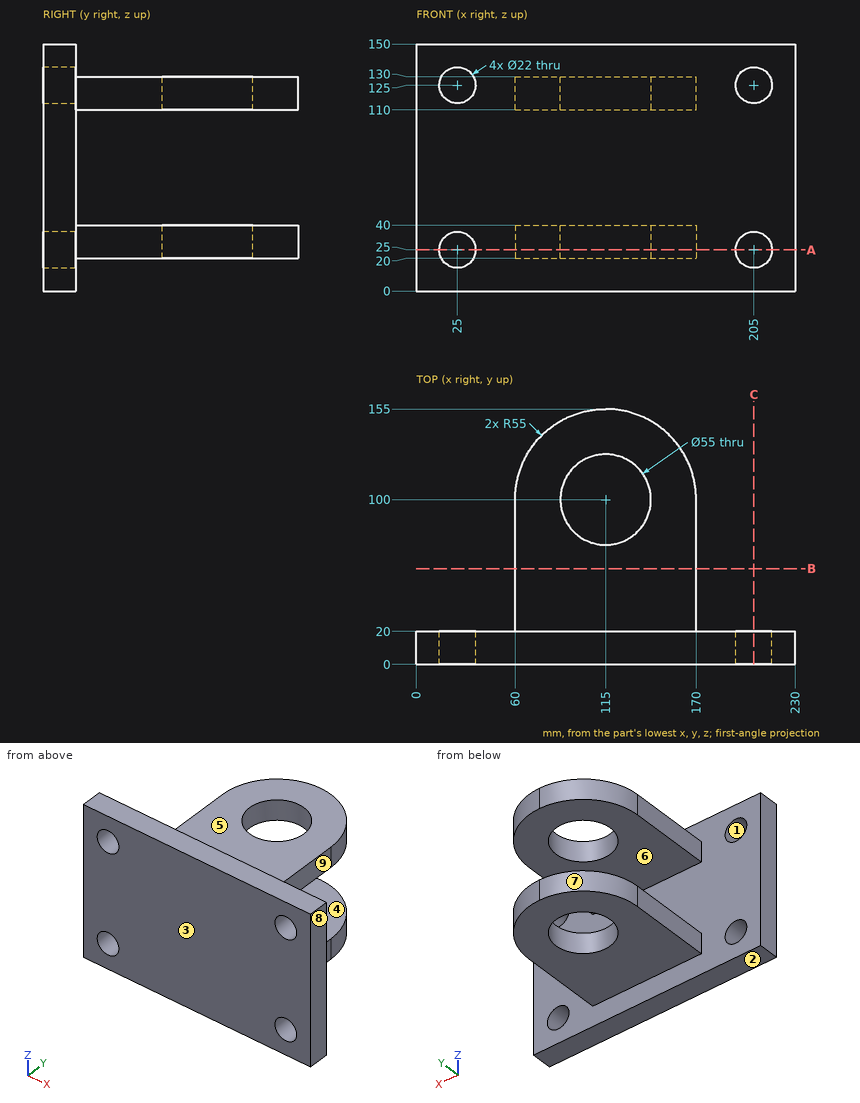
Answer from the drawing. Dimensions are ordinates in mm from the lowest x, y and z of the part. A direction names the side the tool comes from. Give positions to 0.01 mm unless a question says otherwise; leave off trailing zeros. Write each loop counter-clockwise with the first axis right and the second up, starting at its lowest first coordinate (ties: lowest second). Pieces come first, ordered by that corner, then holes. Notation, with made-up numbers: (70.5, 70) - (93.5, 70) arc R37 ccw to (93.5, 108) - close; hole circle Ø7 at (22, 53.5). An arc over 180 degrees is marked (long way). Answer in a Markdown table with one row per item. Add a question column.
Item 1: Section B-B, the plane y = 58 is taken. Write down the section's boundary in (x, z).
Item 2: Find the intervals of material crossed by L1, parallel to X at y = 10, z = 25; L2, parallel to Y at x = 116, z = 29.5; L3, parallel to Z at x = 68, y = 114.5, in increasing order.
Item 3: Section C-C, the plane x = 205 is taken. Write down the section's boundary in (y, z), and give its area (3 significant figures).
Item 4: Flat-ended cylindrical pins translate along their axes: P1, Ø10, axis at y = 79.5, z = 121, coming from the +X side; P2, Ø13, axis at x = 25, z = 25, coming from the -Y side; P3, Ø1, axis at x = 186.5, z = 89, coming from the -Y side; P4, Ø1, axis at x = 109, z = 71.5, coming from the +Y side. Find the tip coordinate at first contact, or state that the pin passes through.
Item 5: Section A-A, the plane z = 25 is taken. Count the separate pieces of the cut face and the enclosed holes in it, and give its area (3 significant figures).
Item 6: A tool of negligible diameter and unlimited length cuts with its end or side. For the marked faces 5, 6, 7, 8 and 9, from which of +Z, -Z, +X, -X, +Y, -Y can it reach the whole face along a straight path? Write none if from no direction.
Item 7: Determine the mould class of the marked faces 1, 2, 3 and 4 for opening direction Z: pulls with the +Z half, pulls with the -Z half, needs draft (parallel to the pull), parting line crosses it, or undercut.
Recorded:
| question | item | result |
|---|---|---|
| 1 | outline | (60, 20) - (170, 20) - (170, 40) - (60, 40) - close; (60, 110) - (170, 110) - (170, 130) - (60, 130) - close |
| 2 | L1 | x = 0 to 14, 36 to 194, 216 to 230 |
| 2 | L2 | y = 0 to 72.52, 127.48 to 154.99 |
| 2 | L3 | z = 20 to 40, 110 to 130 |
| 3 | outline | (0, 0) - (20, 0) - (20, 14) - (0, 14) - close; (0, 36) - (20, 36) - (20, 114) - (0, 114) - close; (0, 136) - (20, 136) - (20, 150) - (0, 150) - close |
| 3 | area | 2,120 mm2 |
| 4 | P1 | stops at x = 170 |
| 4 | P2 | passes through |
| 4 | P3 | stops at y = 0 |
| 4 | P4 | stops at y = 20 |
| 5 | separate pieces | 3 |
| 5 | enclosed holes | 1 |
| 5 | area | 14,900 mm2 |
| 6 | face 5 | +Z, +X, -X, +Y |
| 6 | face 6 | +X, -X, +Y |
| 6 | face 7 | +Z, -Z, -X, +Y |
| 6 | face 8 | +Z, -Z, +X, +Y, -Y |
| 6 | face 9 | +Z, -Z, +X, +Y |
| 7 | face 1 | undercut |
| 7 | face 2 | pulls with the -Z half |
| 7 | face 3 | needs draft |
| 7 | face 4 | undercut |
